Autodesk Inventor part; units mm, degrees
ref_plane "Work Plane1" through (-7.5, 0, 0) normal (-1, 0, 0) x (0, 0, 1)
ref_plane "YZ Plane" through (0, 0, 0) normal (1, 0, 0) x (0, 1, 0)
ref_plane "XZ Plane" through (0, 0, 0) normal (0, 1, 0) x (-1, 0, 0)
sketch "Sketch1" plane through (0, 0, 0) normal (0, 0, 1) x (1, 0, 0)
  line L0 (0, 0) -> (-15, 0)
  line L1 (-15, 0) -> (-15, 15)
  line L2 (-15, 15) -> (0, 15)
  line L3 (0, 15) -> (0, 0)
  dimension "d0" = 15
  dimension "d1" = 15
extrude "Extrusion1" add sketch "Sketch1" along normal blind 26
sketch "Sketch2" plane through (0, 0, 26) normal (0, 0, 1) x (1, 0, 0)
  circle A0 centre (-7.5819, 7.5) radius 7
  point P0 (0, 0)
  dimension "d4" = 14
extrude "Extrusion2" add sketch "Sketch2" along normal blind 5
sketch "Sketch3" plane through (-7.5819, 7.5, 31) normal (0, 0, 1) x (1, 0, 0)
  line L0 (-5, 5) -> (5, 5)
  line L1 (5, 5) -> (5, -5)
  line L2 (5, -5) -> (-5, -5)
  line L3 (-5, -5) -> (-5, 5)
  line L4 (-5, 5) -> (5, -5) construction
  line L5 (5, 5) -> (-5, -5) construction
  point P0 (7.5819, -7.5)
  point P1 (0, 0)
  dimension "d7" = 10
  dimension "d8" = 10
extrude "Extrusion3" add sketch "Sketch3" along normal blind 12.5
sketch "Sketch4" plane through (0, 0, 0) normal (0, 0, -1) x (-1, 0, 0)
  circle A0 centre (7.5819, 7.5) radius 7
  circle A1 centre (7.5819, 7.5) radius 7
  point P0 (0, 0)
  dimension "d11" = 14
extrude "Extrusion4" add sketch "Sketch4" along normal blind 7.5
sketch "Sketch5" plane through (-7.5819, 7.5, -7.5) normal (0, 0, -1) x (-1, 0, 0)
  line L0 (-5, -5) -> (5, -5)
  line L1 (5, -5) -> (5, 5)
  line L2 (5, 5) -> (-5, 5)
  line L3 (-5, 5) -> (-5, -5)
  line L4 (-5, -5) -> (5, 5) construction
  line L5 (5, -5) -> (-5, 5) construction
  point P0 (-7.5819, -7.5)
  point P1 (0, 0)
  dimension "d14" = 10
  dimension "d15" = 10
extrude "Extrusion5" add sketch "Sketch5" along normal blind 8
ref_plane "Work Plane1" through (-7.5, 0, 0) normal (-1, 0, 0) x (0, 0, 1)
sketch "Sketch6" plane through (-7.5, 0, 0) normal (-1, 0, 0) x (0, 0, 1)
  line L0 (-15.5, 12.5) -> (-15.5, 2.5)
  line L1 (-7.5, 2.5) -> (-15.5, 2.5)
  arc A0 (-15.5, 2.5) -> (-16.5, 2.5) centre (-16, 2.5) ccw
  line L2 (-28.5, 2.5) -> (-16.5, 2.5)
  arc A1 (-30.0167, 7.5) -> (-28.5, 2.5) centre (-21.0167, 7.5) ccw
  line L3 (-30.0167, 7.5) -> (-15.5, 7.5)
  line L4 (-15.5, 2.5) -> (-15.5, 7.5)
  point P0 (0, 0)
  dimension "d19" = 0.5
  dimension "d20" = 1
  dimension "d21" = 12
  dimension "d22" = 18
revolve "Revolution1" add sketch "Sketch6" angle 360 about axis through (-7.5, 7.5, -30.0167) along (0, 0, 1)
sketch "Sketch7" plane through (-15, 0, 0) normal (-1, 0, 0) x (0, 0, 1)
  line L0 (0, 15) -> (26, 15)
  line L1 (0, 15) -> (0, 0)
  point P0 (6, 7.5)
  dimension "d31" = 7.5
  dimension "d32" = 6
hole "Hole1" at (-15, 7.5, 6) direction (1, 0, 0) diameter 3 end through all
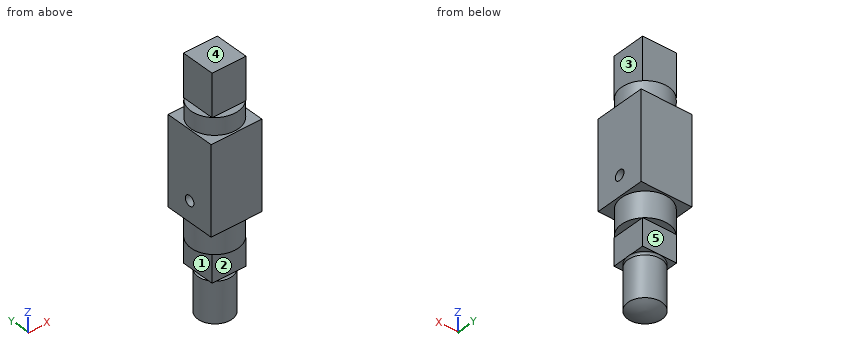
Could you check a few things on this model? Use its own coordinates, in mm. Face numbers are marked on the shaded views. A direction names the side the tool comes from. Round coordinates to 2 decimals unless told otherwise and drop trailing zeros. Loops run counter-clockwise (first coordinate to the right, second up) from the corner with the lowest first, then second, coordinate; pieces in that order, holes last.
Q1. For P1, Ø5, axis at y = 8.5, z = 37, coming from the +X side; P2, Ø8, axis at x = -8, z = 38, coming from the -Y side; P3, Ø4, axis at y = 3, z = -3, coming from the +X side; P4, Ø3, axis at x = -5.5, y = 2, coming from the +Z side, each with a flat end and sliding along its axis, tell me the tip position at first contact or that it passes through.
Q2. I want a section at C-C (y = 1.5). Write out the boundary of the cut face in (x, z), and give its area (3 significant figures).
Q3. I want a section at B-B (z = 39). Write out the boundary of the cut face in (x, y), and give its area (3 significant figures).
Q4. On a 3-axis mill with a long thin cutter (end or side, diameter ignored), from which of +Z, -Z, +X, -X, +Y, -Y can I reach the whole of each face in a straight line? I mean the marked faces 1, 2 and 3. Say none if no direction works.
Q5. I want a section at D-D (z = -23). Write out the boundary of the cut face in (x, y).
Q6. I want a section at A-A (z = 6). Write out the boundary of the cut face in (x, y), and give its area (3 significant figures).
Q7. Thinking about a two-plate mould opening in Z: for the marked faces 4 and 5, which applies, pulls with the +Z half, pulls with the -Z half, needs draft (parallel to the pull), parting line crosses it, or undercut?
Q8. Please list where these lines run through material, in increasing order: L1, parallel to Y at x = -9.25, z = 6; L2, parallel to Y at x = -4.25, z = -9.5; L3, parallel to Z at x = -9, y = 7.5.
Answer below:
1. P1: stops at x = -2.58
1. P2: stops at y = 2.5
1. P3: stops at x = -1.04
1. P4: stops at z = 43.5
2. outline: (-15, 0) - (-11.19, 0) - (-11.19, -7.5) - (-3.98, -7.5) - (-3.98, 0) - (0, 0) - (0, 26) - (-3.98, 26) - (-3.98, 31) - (-11.19, 31) - (-11.19, 26) - (-15, 26) - close
2. area: 480 mm2
3. outline: (-12.58, 2.5) - (-2.58, 2.5) - (-2.58, 12.5) - (-12.58, 12.5) - close
3. area: 100 mm2
4. face 1: -Z, -X, +Y, -Y
4. face 2: -Z, +X, -X, -Y
4. face 3: +Z, +X, +Y, -Y
5. outline: circle Ø10 at (-7.5, 7.5)
6. outline: (-15, 0) - (0, 0) - (0, 6) - (-15, 6) - close; (-15, 9) - (0, 9) - (0, 15) - (-15, 15) - close
6. area: 180 mm2
7. face 4: pulls with the +Z half
7. face 5: needs draft
8. L1: y = 0 to 6, 9 to 15
8. L2: y = 2.5 to 12.5
8. L3: z = -29.89 to 4.5, 7.5 to 43.5
